For this review, use the dimensioned drawing (mm, ordinates from the lowest corner) and the shaded views. Coordinates: 2 decimals unless noted, no trailing zeros. Order: outer loops, then holes, each group sorted by start corner. A loop starts at its lowest first (then second) coordinate and runs counter-clockwise, first axis right, second up. Notation, with made-up numbers: (46, 88) -> (88, 88) arc R13 ccw to (88, 106) -> close; hole circle Ø3 at (-23, 70). An arc over 180 degrees is marked (long way). Return JSON: item names as keys, results as strings. Group by question number.
Item 1: Take a section at A-A (y = 27). Write out the cut boundary in (x, z) (3 decimals).
Item 2: For line 1 along Y through (x, z) = (35, 1.95); line 2 along Y through (x, z) = (18, 2.4); line 3 along X through (y, z) = (26, 2.65), list the stretches that pass through material, from the lowest coordinate up.
Item 3: Take a section at B-B (z = 0.8). Count the separate pieces of the cut face and the enclosed holes in it, then the cut area to 3 significant figures.
Item 4: Take a section at C-C (x = 91). Write out the cut boundary in (y, z) (3 decimals).
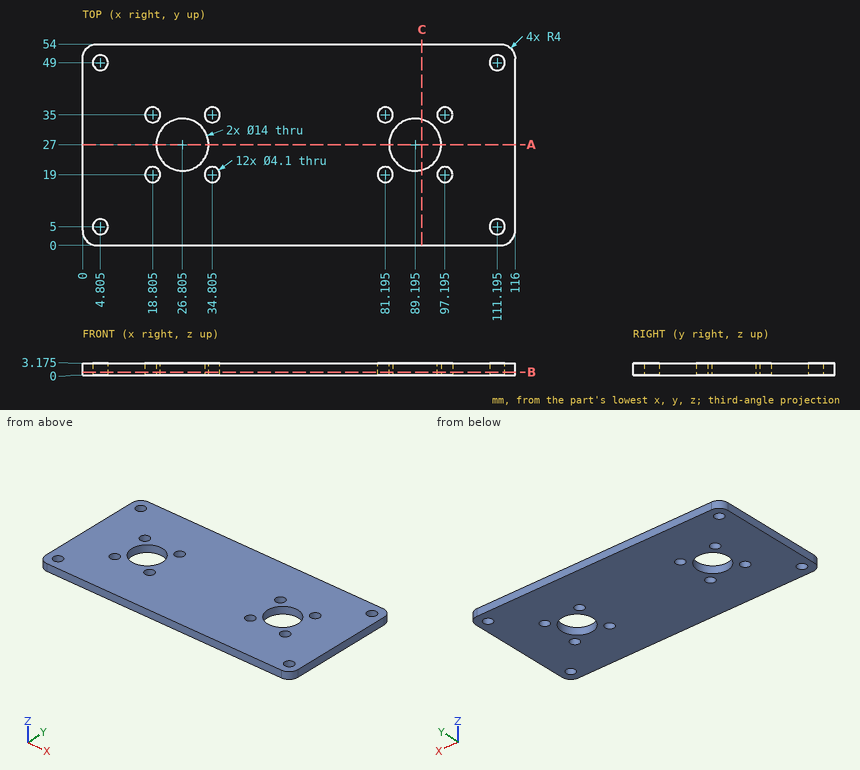
Findings below:
{
 "1": {"outline": "(0, 0) -> (19.805, 0) -> (19.805, 3.175) -> (0, 3.175) -> close; (33.805, 0) -> (82.195, 0) -> (82.195, 3.175) -> (33.805, 3.175) -> close; (96.195, 0) -> (116, 0) -> (116, 3.175) -> (96.195, 3.175) -> close"},
 "2": {"line 1": "y = 0 to 16.96, 21.04 to 32.96, 37.04 to 54", "line 2": "y = 0 to 17.11, 20.89 to 33.11, 36.89 to 54", "line 3": "x = 0 to 19.88, 33.73 to 82.27, 96.12 to 116"},
 "3": {"separate pieces": "1", "enclosed holes": "14", "area": "5,780 mm2"},
 "4": {"outline": "(0, 0) -> (20.237, 0) -> (20.237, 3.175) -> (0, 3.175) -> close; (33.763, 0) -> (54, 0) -> (54, 3.175) -> (33.763, 3.175) -> close"}
}
